Job drawing, mm, ordinate dimensions from the low corner. One solid piece. A direction names the side the tool comes from. Give positions to 0.01 mm unless a question says otherwise; leave off trailing zeros. Order: outer loops, then holes, each group sorted by start corner. A loop starts at its lowest first (then second) coordinate and runs counter-clockwise, first axis right, second up.
Item 1: Band-saw the part on C-C on y = 41. Give the cut face in (x, z) (1 decimal).
Item 2: Band-saw the part on D-D on z = 35. Give the cut face in (x, y) (1 decimal).
Item 3: Wall check: L1, parallel to X at y = 3, z = 13 (1 decimal); L2, parallel to X at y = 42.5, z = 36 (1 decimal); L3, parallel to X at y = 10.5, z = 16.5. Give the ranges that are in metal, low to high.
Item 4: Band-saw the part on A-A on y = 5. Give the cut face in (x, z) (1 decimal).
Item 5: Flat gauge pins, fed straight in: P1, Ø3, axis at x = 31.5, y = 12.5, coming from the +Z side; P2, Ø19.5, axis at x = 57.5, y = 26.5, coming from the +Z side; P3, Ø2, axis at y = 32, z = 24, coming from the -X side; P4, Ø1.5, axis at x = 54, z = 29, coming from the -Y side. Where does each tip first touch, or does it go through?
Item 6: Two-plate mould, pull along X, no slides. Class the marked faces 4, 5, 6 and 7: released by +X, released by -X, zero draft, split by the parting line, or undercut.
Item 7: Band-saw the part on B-B on z = 13. Give the cut face in (x, y) (1 decimal), plus the area to 3 significant figures.
Item 8: Which spindle directions (+Z, -Z, +X, -X, +Y, -Y) get a long thin tool onto all of the face, cutting with end or side? Do the marked faces 1, 2 and 3. Say none if no direction does.
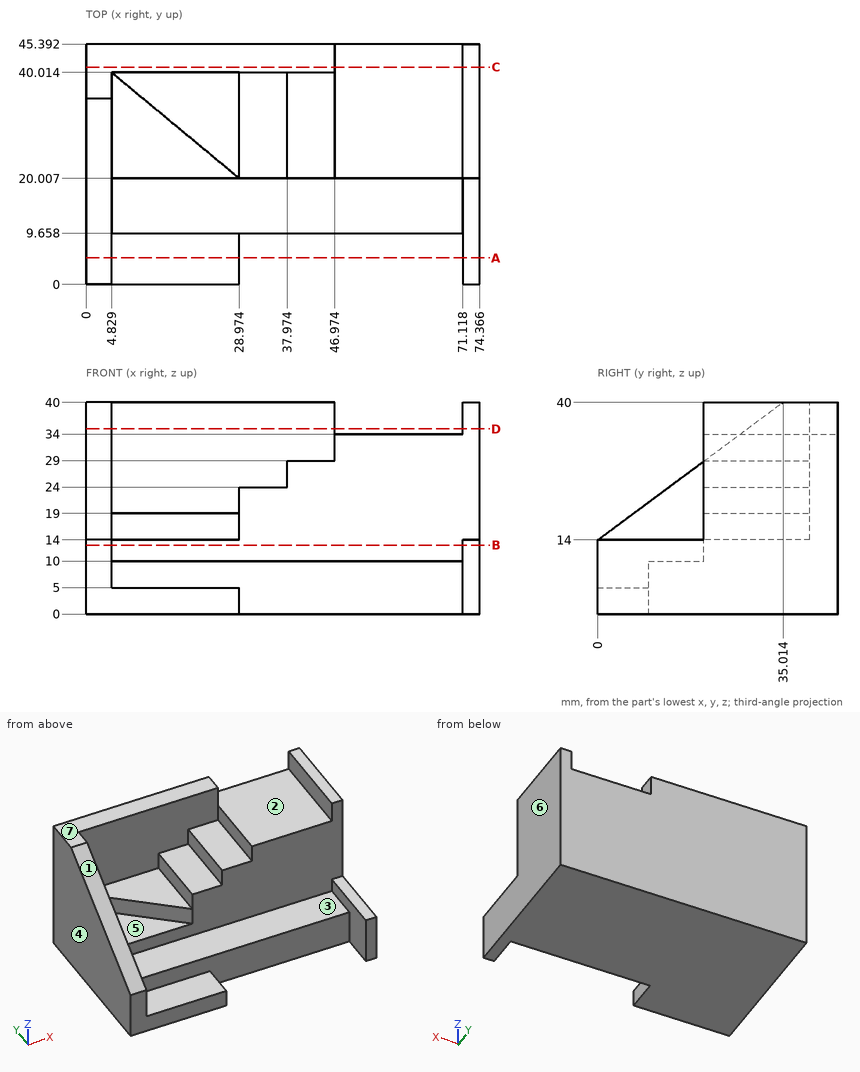
The answers:
1. outline: (0, 0) - (74.4, 0) - (74.4, 40) - (71.1, 40) - (71.1, 34) - (47, 34) - (47, 40) - (0, 40) - close
2. outline: (0, 28.3) - (4.8, 28.3) - (4.8, 40) - (47, 40) - (47, 45.4) - (0, 45.4) - close; (71.1, 20) - (74.4, 20) - (74.4, 45.4) - (71.1, 45.4) - close
3. L1: x = 0 to 4.8, 71.1 to 74.4
3. L2: x = 0 to 47, 71.1 to 74.4
3. L3: x = 0 to 4.83
4. outline: (0, 0) - (29, 0) - (29, 5) - (4.8, 5) - (4.8, 17.7) - (0, 17.7) - close; (71.1, 0) - (74.4, 0) - (74.4, 14) - (71.1, 14) - close
5. P1: stops at z = 10
5. P2: stops at z = 34
5. P3: stops at x = 0
5. P4: stops at y = 20.01
6. face 4: released by -X
6. face 5: undercut
6. face 6: released by +X
6. face 7: zero draft
7. outline: (0, 0) - (4.8, 0) - (4.8, 20) - (71.1, 20) - (71.1, 0) - (74.4, 0) - (74.4, 45.4) - (0, 45.4) - close
7. area: 2,050 mm2
8. face 1: +Z, -X, -Y
8. face 2: +Z, +Y, -Y
8. face 3: +Z, -Y
